Here's how the part is built. I have some questions about the finished solid (model axes, mm). Give positions to 0.01 mm unless a question says otherwise; leave off trailing zeros. Loops run counter-clockwise (first coordinate to the right, second up) from the corner with the lowest first, then second, coordinate; pieces in that order, holes last. Notation, with made-up numbers: (25.25, -35) -> (45.25, -35) arc R24 ccw to (45.25, -2) -> close; hole circle Ø10 at (38, -10.75). An arc over 180 degrees is marked (long way). Answer in a Markdown table with one row per item. Add a question column.
Item 1: If we section it at A-A (x = -2): Write out the boundary of the cut face in (y, z) (3 decimals).
Item 2: If I drill on line 1 (Y direction, x = 118, z = 0) (3 decimals); line 2 (Z direction, x = -33, y = 0.5); line 3 (X direction, y = -0.75, z = -1.5), over which ranges is the centre line in solid material (lowest first)?
Item 3: For P1, Ø1, axis at x = 85, y = -2.5, coming from the +Z side; P2, Ø2, axis at x = 69.5, y = 1.5, coming from the -Z side, each with a flat end and sliding along its axis, tell me the tip position at first contact or that it passes through.
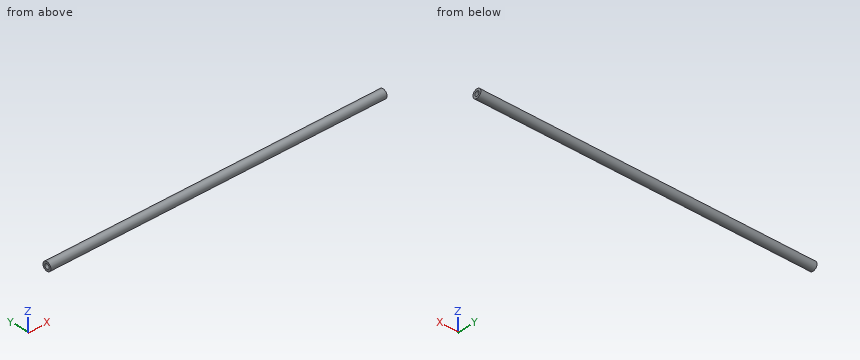
```python
from build123d import *

# Parameters (mm, degrees)
SKETCH1_R           = 3.175
BOSS_EXTRUDE1_DEPTH = 123.19


with BuildPart() as part:
    # Sketch1 → Boss-Extrude1 (new, symmetric)
    with BuildSketch(Plane(origin=(0, 0, 0), x_dir=(0, 0, -1), z_dir=(1, 0, 0))):
        with Locations(Location((0, 0, 0), (0, 0, 180))):
            Circle(SKETCH1_R)
    extrude(amount=BOSS_EXTRUDE1_DEPTH, both=True)

    # Sketch4 → Tap Drill for #8-32 Tap1 (revolve, cut)
    with BuildSketch(Plane(origin=(123.19, 0, 0), x_dir=(0, 0, -1), z_dir=(0, 1, 0))):
        Polygon((0, 0), (0, 11.197806461), (1.7272, 10.16), (1.7272, 0), align=None)
    tap_drill_for_8_32_tap1 = revolve(axis=Axis((129.54, 0, 0), (-1, 0, 0)), mode=Mode.SUBTRACT)

    # Mirror1: Tap Drill for #8-32 Tap1 across plane
    add(tap_drill_for_8_32_tap1.mirror(Plane(origin=(0, 0, 0), x_dir=(0, 0, 1), z_dir=(1, 0, 0))), mode=Mode.SUBTRACT)


solid = part.part
```
Recorded:
| question | item | result |
|---|---|---|
| 1 | outline | circle Ø6.35 at (0, 0) |
| 2 | line 1 | y = -3.175 to -1.727, 1.727 to 3.175 |
| 2 | line 2 | z = -3.14 to 3.14 |
| 2 | line 3 | x = -113 to 113 |
| 3 | P1 | stops at z = 2.47 |
| 3 | P2 | stops at z = -3.14 |
